from build123d import *

# Parameters (mm, degrees)
SKETCH_R        = 2.5
PAD_DEPTH       = 25
SKETCH001_W     = 5
SKETCH001_H     = 0.5
POCKET_DEPTH    = 5
SKETCH002_R     = 1.5
POCKET001_DEPTH = 56.462524


with BuildPart() as part:
    # Sketch → Pad (new body)
    with BuildSketch(Plane.XY):
        Circle(SKETCH_R)
    pad = extrude(amount=PAD_DEPTH)

    # Sketch001 (on Face3 of Pad) → Pocket (cut)
    with BuildSketch(Plane.XY.offset(25)):
        with Locations((0, 2.25)):
            Rectangle(SKETCH001_W, SKETCH001_H)
        with Locations((0, -2.25)):
            Rectangle(SKETCH001_W, SKETCH001_H)
    pocket = extrude(amount=-POCKET_DEPTH, mode=Mode.SUBTRACT)

    # Sketch002 (on Face4 of Pocket) → Pocket001 (cut, through all)
    with BuildSketch(Plane.XZ.offset(2)):
        with Locations((0, 23)):
            Circle(SKETCH002_R)
    pocket001 = extrude(amount=-POCKET001_DEPTH, mode=Mode.SUBTRACT)

    # Mirrored: Pad across face of Pocket001
    add(pad.mirror(Plane(origin=(0, 0, 0), x_dir=(1, 0, 0), z_dir=(0, 0, -1))))

    # Mirrored001: Pocket across XY
    add(pocket.mirror(Plane.XY), mode=Mode.SUBTRACT)

    # Mirrored002: Pocket001 across XY
    add(pocket001.mirror(Plane.XY), mode=Mode.SUBTRACT)


solid = part.part
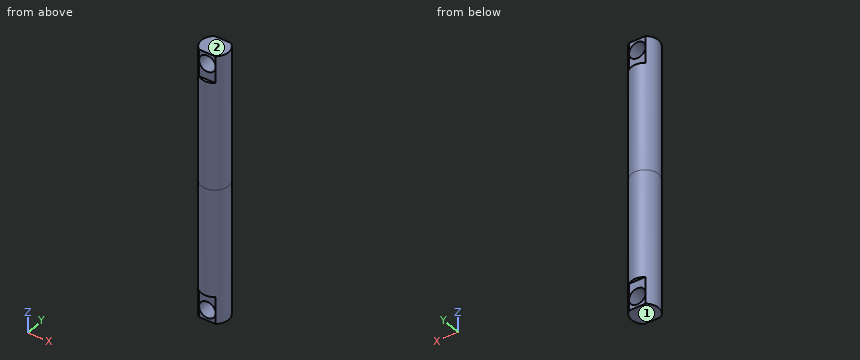
Geometry: final body of the model. Coordinates: model frame, mm. Face numbers are marked on the shaded views. Give positions to 0.01 mm unless a question says otherwise; leave off trailing zeros. Order: outer loops, then holes, each group sorted by start corner. A loop starts at its lowest first (then second) coordinate and runs counter-clockwise, first axis right, second up. Notation, with made-up numbers: (17.25, 22.25) -> (63.25, 22.25) arc R19 ccw to (63.25, 52.25) -> close; hole circle Ø8 at (-30, 86.25). An arc over 180 degrees is marked (long way). Answer as a JSON object with one key per item and string values.
Q1. First-contact query: pin 1 (0.9 mm diameter, centred on x = 0.5, z = -22, fed in from +Y); pin 2 (1.5 mm diameter, centred on x = 1.5, z = -18, fed in from +Y); pin 3 (2 mm diameter, centred on x = 0.5, z = 23.5, fed in from -Y); pin 4 (2.5 mm diameter, centred on x = 0, z = 23, fed in from -Y). Flat tips, straight axial feed; report the tip coordinate or a pass-through.
Entries:
{"pin 1": "stops at y = 2", "pin 2": "stops at y = 2.38", "pin 3": "stops at y = -2", "pin 4": "passes through"}
Q2. Section A-A (x = 0). Output: boundary loops of the cut face in (y, z), plus the area to 3 significant figures.
Entries:
{"outline": "(-2.5, -20) -> (-2, -20) -> (-2, -21.5) -> (2, -21.5) -> (2, -20) -> (2.5, -20) -> (2.5, 20) -> (2, 20) -> (2, 21.5) -> (-2, 21.5) -> (-2, 20) -> (-2.5, 20) -> close; (-2, -25) -> (2, -25) -> (2, -24.5) -> (-2, -24.5) -> close; (-2, 24.5) -> (2, 24.5) -> (2, 25) -> (-2, 25) -> close", "area": "216 mm^2"}
Q3. Section B-B (y = 0). Output: boundary loops of the cut face in (x, z), plus the area to 3 significant figures.
Entries:
{"outline": "(-2.5, -25) -> (2.5, -25) -> (2.5, 25) -> (-2.5, 25) -> close; hole circle Ø3 at (0, -23); hole circle Ø3 at (0, 23)", "area": "236 mm^2"}
Q4. Section C-C (z = 6). Output: boundary loops of the cut face in (x, y).
Entries:
{"outline": "circle Ø5 at (0, 0)"}
Q5. Material intervals for probe 1 along Z at (x, y) = (0, 0.7); probe 2 along Z at (x, y) = (-1.3, -1.95); probe 3 along X at (y, z) = (0, 23), sorted ascending.
Entries:
{"probe 1": "z = -25 to -24.5, -21.5 to 21.5, 24.5 to 25", "probe 2": "z = -25 to -23.75, -22.25 to 22.25, 23.75 to 25", "probe 3": "x = -2.5 to -1.5, 1.5 to 2.5"}
Q6. Draft query along Z for the marked faces 1 and 2. Return one class per face: released by +Z, released by -Z, zero draft, split by the parting line, or undercut.
Entries:
{"face 1": "released by -Z", "face 2": "released by +Z"}
